Input: part model. Units: mm. Frame: model coordinates. A direction names the side the tool comes from. Coordinates: 2 decimals unless noted, no trailing zeros. Order: outer loops, then holes, each group sorted by start corner. A loop starts at its lowest first (then second) coordinate and runs counter-clockwise, first axis right, second up. Notation, with made-up numbers: (27.25, -7.5) -> (81.25, -7.5) arc R11 cw to (81.25, 5.5) -> close; hole circle Ø4 at (33.5, 8.25). An arc over 180 degrees is marked (long way). One line per item, written item: value. Start each with the question number.
from build123d import *

# Parameters (mm, degrees)
SKETCH5_W           = 100
SKETCH5_H           = 50
SKETCH5_R           = 4
BOSS_EXTRUDE6_DEPTH = 10
SKETCH6_W           = 125
SKETCH6_H           = 50
SKETCH6_R           = 4
BOSS_EXTRUDE7_DEPTH = 10
SKETCH7_W           = 125
SKETCH7_H           = 50
SKETCH7_R           = 4
BOSS_EXTRUDE8_DEPTH = 10


with BuildPart() as part:
    # Sketch5 → Boss-Extrude6 (new body)
    with BuildSketch(Plane(origin=(0, 0, 0), x_dir=(0, 0, -1), z_dir=(1, 0, 0))):
        Rectangle(SKETCH5_W, SKETCH5_H)
        Circle(SKETCH5_R, mode=Mode.SUBTRACT)
    extrude(amount=-BOSS_EXTRUDE6_DEPTH)

    # Sketch6 → Boss-Extrude7 (add)
    with BuildSketch(Plane(origin=(0, 0, -50), x_dir=(-1, 0, 0), z_dir=(0, 0, -1))):
        with Locations((62.5, 0)):
            Rectangle(SKETCH6_W, SKETCH6_H)
        with Locations((62.5, 0)):
            Circle(SKETCH6_R, mode=Mode.SUBTRACT)
    extrude(amount=-BOSS_EXTRUDE7_DEPTH)

    # Sketch7 → Boss-Extrude8 (add)
    with BuildSketch(Plane.XY.offset(50)):
        with Locations((-62.5, 0)):
            Rectangle(SKETCH7_W, SKETCH7_H)
        with Locations((-62.5, 0)):
            Circle(SKETCH7_R, mode=Mode.SUBTRACT)
    extrude(amount=-BOSS_EXTRUDE8_DEPTH)


solid = part.part
1) Ray query, line 1 along Z through (x, y) = (-119, -14); line 2 along Y through (x, z) = (-62, -45); line 3 along X through (y, z) = (2, 6). Return the intervals inside material, ascending. Write a range as from..to.
2) Section query C-C, the plane z = 0. Return the cut outline in (x, y), plus the area to 3 significant figures.
3) Access query for faces 4 (the flat face through (-68, 0, 40)), 5 (the flat face through (-49, 25, -41)). Directions: +Z, -Z, +X, -X, +Y, -Y. A direction counts if a zero-diameter tool reaches every point of the face in a straight line with its end or side. Return the directions, or none.
4) Mould query, pull axis Z, two halves, no side actions, for faces 1 (the flat face through (-62, -6, -50)), 2 (the cylindrical face through (-4.93, -3.905, 0.867)), 3 (the flat face through (0, 6, 1)). Classes: +Z half, -Z half, draft (parallel to the pull), parting line (faces both ways), or undercut.
5) Section query B-B, the plane x = -112. Return the cut outline in (y, z).
6) Pin query (flat end, axial travel): pin 1 Ø9 at (x, y) = (-62.5, 0) entering from +Z; pin 2 Ø6.5 at (y, z) = (0, 0) entering from -X; pin 3 Ø2 at (y, z) = (-9.5, -17.5) entering from -X. Return the tip coordinate at first contact, or that it passes through.
7) Section query A-A, the plane x = -62.5. Return the cut outline in (y, z), plus the area to 3 significant figures.
8) Section query D-D, the plane y = 14. Return the cut outline in (x, z).
Entries:
1. line 1: z = -50..-40, 40..50
1. line 2: y = -25..-3.97, 3.97..25
1. line 3: x = -10..0
2. outline: (-10, -25) -> (0, -25) -> (0, -4) -> (-10, -4) -> close; (-10, 4) -> (0, 4) -> (0, 25) -> (-10, 25) -> close
2. area: 420 mm2
3. face 4: -X, +Y, -Y
3. face 5: +Z, -Z, +X, -X, +Y
4. face 1: -Z half
4. face 2: undercut
4. face 3: draft
5. outline: (-25, -50) -> (25, -50) -> (25, -40) -> (-25, -40) -> close; (-25, 40) -> (25, 40) -> (25, 50) -> (-25, 50) -> close
6. pin 1: stops at z = 50
6. pin 2: passes through
6. pin 3: stops at x = -10
7. outline: (-25, -50) -> (-4, -50) -> (-4, -40) -> (-25, -40) -> close; (-25, 40) -> (-4, 40) -> (-4, 50) -> (-25, 50) -> close; (4, -50) -> (25, -50) -> (25, -40) -> (4, -40) -> close; (4, 40) -> (25, 40) -> (25, 50) -> (4, 50) -> close
7. area: 840 mm2
8. outline: (-125, -50) -> (0, -50) -> (0, 50) -> (-125, 50) -> (-125, 40) -> (-10, 40) -> (-10, -40) -> (-125, -40) -> close
